Read the model definition and answer for the solid it produces. Units are mm, in the model's axes. A direction names the side the tool comes from. Coordinates: 2 decimals unless noted, no trailing zeros. Order: outer loops, then holes, each group sorted by start corner. A loop starts at its lowest first (then second) coordinate and runs counter-clockwise, first axis right, second up. Notation, with made-up numbers: (51.25, 39.25) -> (101.25, 39.25) arc R19 cw to (101.25, 75.25) -> close; hole circle Ø3 at (-3.5, -19). An arc over 180 degrees is marked (long way). Answer in a Markdown table with one row per item.
from build123d import *

# Parameters (mm, degrees)
F0_W     = 63.5
F0_H     = 203.2
F0_W_2   = 12.7
F0_H_2   = 12.7
F1_DEPTH = 19.05
F3_D     = 6.35
F3_DEPTH = 38.1
F3_TIP   = 1.9077324654
F5_D     = 6.35
F5_DEPTH = 38.1
F5_TIP   = 1.9077324654


with BuildPart() as f1:
    # F0 (on Top) → F1 (new body)
    with BuildSketch(Plane.XY):
        Rectangle(F0_W, F0_H)
        Rectangle(F0_W_2, F0_H_2, mode=Mode.SUBTRACT)
    extrude(amount=F1_DEPTH)

    # F3
    with Locations(Plane.XZ.offset(101.6)):
        with Locations((-21.59, 9.525), (21.59, 9.525)):
            Hole(F3_D / 2, depth=F3_DEPTH)
            with Locations((0, 0, -(F3_DEPTH + F3_TIP / 2))):  # 118° drill point
                Cone(0, F3_D / 2, F3_TIP, mode=Mode.SUBTRACT)

    # F5
    with Locations(Plane(origin=(0, 101.6, 0), x_dir=(-1, 0, 0), z_dir=(0, 1, 0))):
        with Locations((21.59, 9.525), (-21.59, 9.525)):
            Hole(F5_D / 2, depth=F5_DEPTH)
            with Locations((0, 0, -(F5_DEPTH + F5_TIP / 2))):  # 118° drill point
                Cone(0, F5_D / 2, F5_TIP, mode=Mode.SUBTRACT)


solid = f1.part
Q1. The part is cut by section A-A (x = 4). Write down the section's boundary in (y, z).
Outcome:
| item | result |
|---|---|
| outline | (-101.6, 0) -> (-6.35, 0) -> (-6.35, 19.05) -> (-101.6, 19.05) -> close; (6.35, 0) -> (101.6, 0) -> (101.6, 19.05) -> (6.35, 19.05) -> close |
Q2. Given pin 1 (5.5 mm diameter, centred on x = 21.59, z = 9.525, fed in from -Y), flat-ended and moving along its own axis, determine where the tip first touches the part or whether it passes through.
Outcome:
| item | result |
|---|---|
| pin 1 | y = -63.24 |
Q3. Consider line 1 (X direction, y = 90, z = 9.5); line 2 (X direction, y = 83, z = 11); line 3 (Z direction, x = 21.59, y = -74.5). Determine where each line is inside the solid, lowest interval first.
Outcome:
| item | result |
|---|---|
| line 1 | -31.75 to -24.76, -18.42 to 18.42, 24.76 to 31.75 |
| line 2 | -31.75 to -24.4, -18.78 to 18.78, 24.4 to 31.75 |
| line 3 | 0 to 6.35, 12.7 to 19.05 |
Q4. For a pull along X with two mould halves and no side action, classify faces 1 (the face through (-18.56, 82.28, 10.48)), 2 (the face through (-31.75, -1, 9)), 3 (the face through (7, 1, 0)) as pulls with the +X half, pulls with the -X half, needs draft (parallel to the pull), parting line crosses it, or undercut.
Outcome:
| item | result |
|---|---|
| face 1 | undercut |
| face 2 | pulls with the -X half |
| face 3 | needs draft |
Q5. For faces 4 (the face through (-24.62, -82.28, 10.48)), 5 (the face through (24.62, 82.28, 10.48)), 6 (the face through (0, -6.35, 9)), determine the directions among +Z, -Z, +X, -X, +Y, -Y from which every point of the face is accessible in a straight line to the end or side of a thin tool.
Outcome:
| item | result |
|---|---|
| face 4 | -Y |
| face 5 | +Y |
| face 6 | +Z, -Z |
